from build123d import *

# Parameters (mm, degrees)
SKETCH_1_R      = 1.5
EXTRUDE_1_DEPTH = 2


with BuildPart() as part:
    # 草图1 → 凸台-拉伸1 (new body)
    with BuildSketch(Plane.XY):
        with BuildLine():
            Line((18.317061038, 8.799028027), (16.317061038, 8.799028027))
            Line((16.317061038, 8.799028027), (16.317061038, 9.733577366))
            ThreePointArc((16.317061038, 9.733577366), (15.251610376, 9.733577366), (15.251610376, 10.799028027))
            Line((15.251610376, 10.799028027), (-8.682938962, 10.799028027))
            Line((-8.682938962, 10.799028027), (-8.682938962, 8.799028027))
            Line((-8.682938962, 8.799028027), (-10.682938962, 8.799028027))
            Line((-10.682938962, 8.799028027), (-10.682938962, 3.799028027))
            Line((-10.682938962, 3.799028027), (-8.682938962, 3.799028027))
            Line((-8.682938962, 3.799028027), (-8.682938962, 0.299028027))
            Line((-8.682938962, 0.299028027), (-6.182938962, 0.299028027))
            Line((-6.182938962, 0.299028027), (-6.182938962, 1.799028027))
            Line((-6.182938962, 1.799028027), (-3.582938962, 1.799028027))
            Line((-3.582938962, 1.799028027), (-3.582938962, 0.299028027))
            Line((-3.582938962, 0.299028027), (-0.582938962, 0.299028027))
            Line((-0.582938962, 0.299028027), (-0.582938962, -2.700971973))
            Line((-0.582938962, -2.700971973), (-3.582938962, -2.700971973))
            Line((-3.582938962, -2.700971973), (-3.582938962, -4.200971973))
            Line((-3.582938962, -4.200971973), (-6.182938962, -4.200971973))
            Line((-6.182938962, -4.200971973), (-6.182938962, -2.700971973))
            Line((-6.182938962, -2.700971973), (-8.682938962, -2.700971973))
            Line((-8.682938962, -2.700971973), (-8.682938962, -6.200971973))
            Line((-8.682938962, -6.200971973), (-10.682938962, -6.200971973))
            Line((-10.682938962, -6.200971973), (-10.682938962, -11.200971973))
            Line((-10.682938962, -11.200971973), (-8.682938962, -11.200971973))
            Line((-8.682938962, -11.200971973), (-8.682938962, -15.200971973))
            Line((-8.682938962, -15.200971973), (3.411134121, -15.200971973))
            Line((3.411134121, -15.200971973), (3.817061038, -15.955763704))
            Line((3.817061038, -15.955763704), (4.222987954, -15.200971973))
            Line((4.222987954, -15.200971973), (16.317061038, -15.200971973))
            Line((16.317061038, -15.200971973), (16.317061038, -11.200971973))
            Line((16.317061038, -11.200971973), (18.317061038, -11.200971973))
            Line((18.317061038, -11.200971973), (18.317061038, -6.200971973))
            Line((18.317061038, -6.200971973), (16.317061038, -6.200971973))
            Line((16.317061038, -6.200971973), (16.317061038, -2.700971973))
            Line((16.317061038, -2.700971973), (13.817061038, -2.700971973))
            Line((13.817061038, -2.700971973), (13.817061038, -4.200971973))
            Line((13.817061038, -4.200971973), (11.217061038, -4.200971973))
            Line((11.217061038, -4.200971973), (11.217061038, -2.700971973))
            Line((11.217061038, -2.700971973), (8.217061038, -2.700971973))
            Line((8.217061038, -2.700971973), (8.217061038, 0.299028027))
            Line((8.217061038, 0.299028027), (11.217061038, 0.299028027))
            Line((11.217061038, 0.299028027), (11.217061038, 1.799028027))
            Line((11.217061038, 1.799028027), (13.817061038, 1.799028027))
            Line((13.817061038, 1.799028027), (13.817061038, 0.299028027))
            Line((13.817061038, 0.299028027), (16.317061038, 0.299028027))
            Line((16.317061038, 0.299028027), (16.317061038, 3.799028027))
            Line((16.317061038, 3.799028027), (18.317061038, 3.799028027))
            Line((18.317061038, 3.799028027), (18.317061038, 8.799028027))
        make_face()
        with Locations((3.817061038, -6.200971973)):
            Circle(SKETCH_1_R, mode=Mode.SUBTRACT)
        with Locations((3.817061038, 3.799028027)):
            Circle(SKETCH_1_R, mode=Mode.SUBTRACT)
        with Locations((3.817061038, -12.192801434)):
            Circle(SKETCH_1_R, mode=Mode.SUBTRACT)
        with BuildLine():
            Line((13.217061038, -13.342801434), (7.917061038, -13.342801434))
            ThreePointArc((7.917061038, -13.342801434), (7.440715441, -12.192801434), (7.917061038, -11.042801434))
            Line((7.917061038, -11.042801434), (13.217061038, -11.042801434))
            Line((13.217061038, -11.042801434), (13.217061038, -13.342801434))
        make_face(mode=Mode.SUBTRACT)
        with BuildLine():
            Line((-5.582938962, -11.042801434), (-0.282938962, -11.042801434))
            ThreePointArc((-0.282938962, -11.042801434), (0.193406634, -12.192801434), (-0.282938962, -13.342801434))
            Line((-0.282938962, -13.342801434), (-5.582938962, -13.342801434))
            Line((-5.582938962, -13.342801434), (-5.582938962, -11.042801434))
        make_face(mode=Mode.SUBTRACT)
    extrude(amount=EXTRUDE_1_DEPTH)


solid = part.part
Geometry check sheet. Reference: the model listing, model coordinates, mm. A direction names the side the tool comes from. Round coordinates to 2 decimals unless told otherwise and drop trailing zeros. Order: outer loops, then holes, each group sorted by start corner. A loop starts at its lowest first (then second) coordinate and runs counter-clockwise, first axis right, second up. Notation, with made-up numbers: (50, 81) -> (83, 81) arc R9 cw to (83, 85) -> close; hole circle Ø1 at (-8.5, 34). An arc over 180 degrees is marked (long way). Use one line per item in the form item = value.
1. Set-up check for faces 4 (the face through (-7, -2.701, 1)), 5 (the face through (11, -11.043, 1)), 6 (the face through (17, -6.201, 1)): record each of +Z, -Z, +X, -X, +Y, -Y from which the full face is reachable in a straight line by a thin tool's end or side.
Working result:
face_4 = +Z, -Z, -X
face_5 = +Z, -Z
face_6 = +Z, -Z, +X
2. Cross-section at D-D, the plane x = 16. Enter the section's corners in (y, z).
Working result:
outline = (-15.2, 0) -> (-2.7, 0) -> (-2.7, 2) -> (-15.2, 2) -> close; (0.3, 0) -> (9.54, 0) -> (9.54, 2) -> (0.3, 2) -> close
3. Cross-section at A-A, the plane y = 1.25. Enter the section's corners in (x, z).
Working result:
outline = (-8.68, 0) -> (-6.18, 0) -> (-6.18, 2) -> (-8.68, 2) -> close; (-3.58, 0) -> (11.22, 0) -> (11.22, 2) -> (-3.58, 2) -> close; (13.82, 0) -> (16.32, 0) -> (16.32, 2) -> (13.82, 2) -> close
4. Scan lines: line 1 along X through (y, z) = (-3, 1.6); line 2 along Y through (x, z) = (11, 1.1); line 3 along Y through (x, z) = (-7.75, 1.25). Record each from-to range of solid material in increasing order. Write a range as from..to.
Working result:
line_1 = -8.68..-6.18, -3.58..11.22, 13.82..16.32
line_2 = -15.2..-13.34, -11.04..-2.7, 0.3..10.8
line_3 = -15.2..-2.7, 0.3..10.8
5. Cross-section at C-C, the plane y = -11.75. Enter the section's corners in (x, z).
Working result:
outline = (-8.68, 0) -> (-5.58, 0) -> (-5.58, 2) -> (-8.68, 2) -> close; (0.13, 0) -> (2.38, 0) -> (2.38, 2) -> (0.13, 2) -> close; (5.25, 0) -> (7.5, 0) -> (7.5, 2) -> (5.25, 2) -> close; (13.22, 0) -> (16.32, 0) -> (16.32, 2) -> (13.22, 2) -> close
6. Go/stop test with flat-tipped pins: pin 1 (0.6 mm diameter, centred on x = 0, z = 1.5, fed in from -Y); pin 2 (1 mm diameter, centred on y = -5, z = 1, fed in from +X); pin 3 (1 mm diameter, centred on y = -1, z = 0.5, fed in from +X). Record where each tip stops, or that it passes through.
Working result:
pin_1 = -15.2
pin_2 = 16.32
pin_3 = 8.22
7. Cross-section at B-B, the plane x = -4. Enter the section's corners in (y, z).
Working result:
outline = (-15.2, 0) -> (-13.34, 0) -> (-13.34, 2) -> (-15.2, 2) -> close; (-11.04, 0) -> (-4.2, 0) -> (-4.2, 2) -> (-11.04, 2) -> close; (1.8, 0) -> (10.8, 0) -> (10.8, 2) -> (1.8, 2) -> close
8. Mould release check, pull along Y, two halves, no side actions. Record for faces 1 (the face through (-10.683, 6, 1)), 2 (the face through (-10, 3.799, 1)), 3 (the face through (17, 8.799, 1)): pulls with the +Y half, pulls with the -Y half, needs draft (parallel to the pull), parting line crosses it, or undercut.
Working result:
face_1 = needs draft
face_2 = undercut
face_3 = pulls with the +Y half
